Can you work these out from the drawing? Everything is in mm from the part's minimum corner. A direction names the side the tool comes from. Round coordinates to 2 decimals unless told otherwise and drop trailing zeros. Order: outer loops, then holes, each group sorted by start corner. A loop starts at its lowest first (then second) coordinate and runs counter-clockwise, first axis right, second up. Notation, with made-up numbers: (8.5, 8.5) - (25.5, 8.5) arc R25 ccw to (25.5, 45.5) - close; hole circle Ø8 at (44, 26). An arc over 180 degrees is marked (long way). Answer as a JSON object with one key per item and string values.
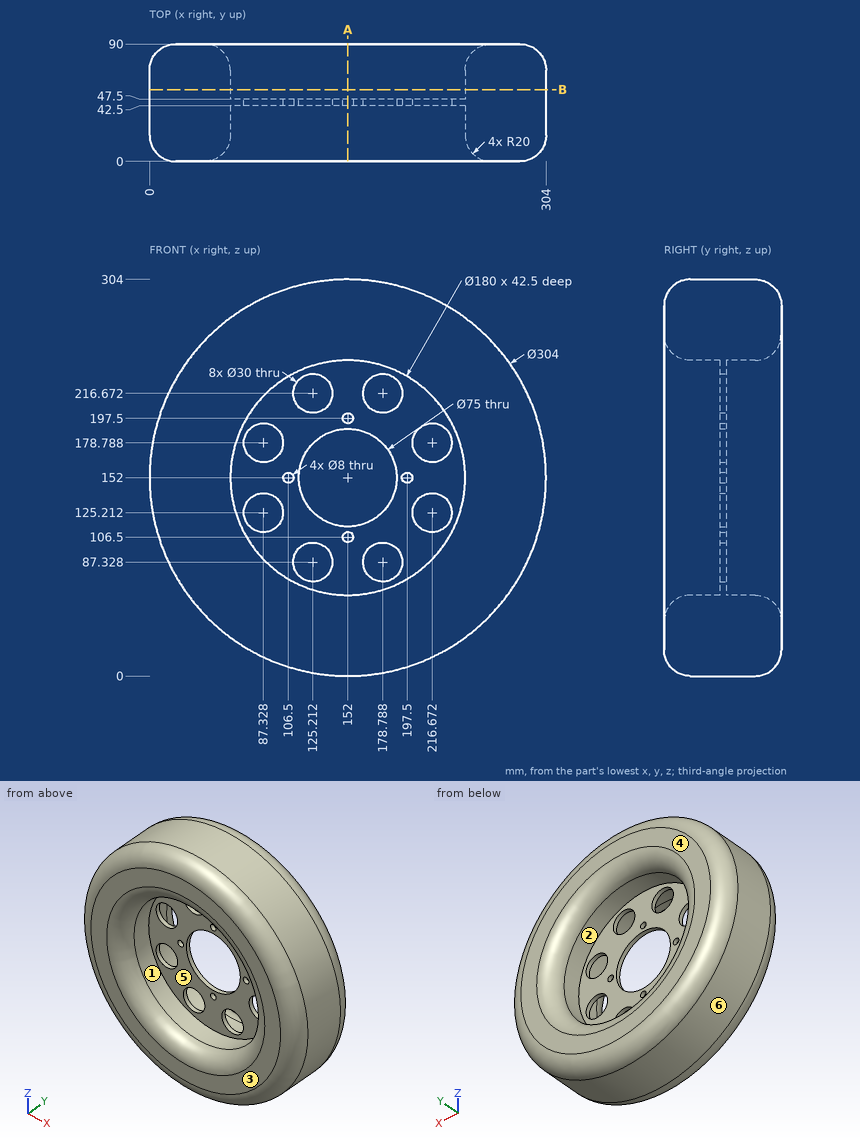
1. For the marked faces 1, 2 and 3, which set-ups out of +Z, -Z, +X, -X, +Y, -Y let a thin tool reach every point of the face, with its end or its side?
Responses:
{"face 1": "-Y", "face 2": "+Y", "face 3": "+Z, -Z, +X, -X, -Y"}
2. Imagine slicing it at B-B (y = 55). List the corners of the cut face in (x, z) for me.
Responses:
{"outline": "circle Ø304 at (152, 152); hole circle Ø180 at (152, 152)"}
3. Imagine slicing it at A-A (x = 152). Give the number of separate pieces and of enclosed holes in the cut face, plus the area to 3 significant figures.
Responses:
{"separate pieces": "4", "enclosed holes": "0", "area": "10,900 mm2"}
4. If I drill on L1, parallel to Z at x = 152, y = 43.9; L2, parallel to Z at x = 209, y = 66.5; L3, parallel to Z at x = 92, y = 42 (1 decimal), over which ranges is the centre line in solid material (lowest first)? Write a range as [from, to].
Responses:
{"L1": "[0, 102.5], [110.5, 114.5], [189.5, 193.5], [201.5, 304]", "L2": "[11.09, 82.35], [221.65, 292.91]", "L3": "[12.3, 84.9], [219.1, 291.7]"}
5. For P1, Ø1, axis at y = 14, z = 195, coming from the +X side; P2, Ø10, axis at x = 115, z = 171.5, coming from the -Y side; P3, Ø12, axis at x = 238.5, z = 110.5, coming from the -Y side, each with a flat end and sliding along its axis, tell me the tip position at first contact or that it passes through.
Responses:
{"P1": "x = 297.05", "P2": "y = 42.5", "P3": "y = 1.7"}
6. Thinking about a two-plate mould opening in Z: for the marked faces 4, 5 and 6, which applies, pulls with the +Z half, pulls with the -Z half, needs draft (parallel to the pull), parting line crosses it, or undercut?
Responses:
{"face 4": "needs draft", "face 5": "undercut", "face 6": "parting line crosses it"}
